Check sheet for the modelled part. Datum: model origin and axes. Units: mm. Coordinates: 2 decimals unless noted, no trailing zeros. Write each loop counter-clockwise with the first axis right and the second up, starting at its lowest first coordinate (ties: lowest second). Pieces come first, ordered by that corner, then holes. Notation, with made-up numbers: M 38.5,35.5 L 45.5,35.5 A20 cw 45.5,71.5 Z; hole C -18,-19 d10. An arc over 180 degrees is marked long. Answer as CSV lines item,"result". Start each with the question number.
Q1. Sectioned sample at D-D, the plane y = 46. Record the cut outline in (x, z), then the cut area to 3 significant figures.
Q2. Sectioned sample at A-A, the plane z = -1.05. Count the separate pieces of the cut face and the enclosed holes in it, then the cut area to 3 significant figures.
Q3. Depth check by flat-ended pin: pin 1 Ø3.5 at (x, y) = (0, 59.309) entering from +Z. Enter the tip coordinate at first touch or a pass-through.
Q4. Sectioned sample at B-B, the plane x = -1. Record the cut outline in (y, z).
Q5. Sectioned sample at C-C, the plane y = -1. Record the cut outline in (x, z), then the cut area to 3 significant figures.
Q6. Thickness scan on line 1 along Y through (x, z) = (0, 0.75) (3 decimals); line 2 along X through (y, z) = (72, -0.1); line 3 along Y through (x, z) = (-0.75, -0.4). Record the ranges inside material, lowest first. Write a range as from..to.
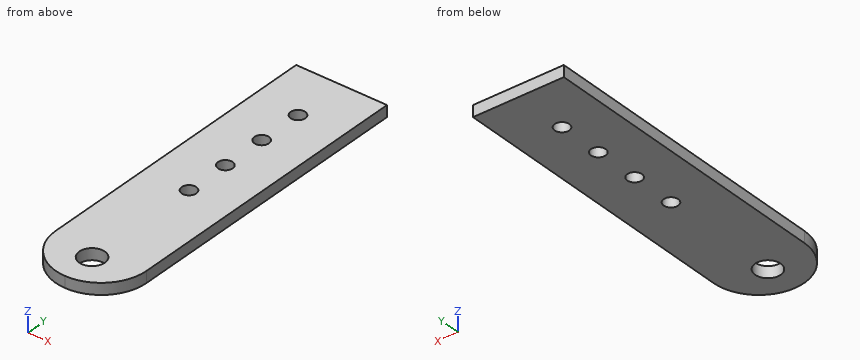
Autodesk Inventor part; units mm, degrees
ref_plane "YZ Plane" through (0, 0, 0) normal (1, 0, 0) x (0, 1, 0)
ref_plane "XZ Plane" through (0, 0, 0) normal (0, 1, 0) x (-1, 0, 0)
ref_plane "XY Plane" through (0, 0, 0) normal (0, 0, 1) x (1, 0, 0)
sketch "Sketch1" plane through (0, 0, 0) normal (0, 0, 1) x (1, 0, 0)
  circle A0 centre (0, 0) radius 3.5687
  line L0 (-12.7, 61.849) -> (12.7, 61.849)
  line L1 (12.7, 61.849) -> (12.7, -9.525)
  line L2 (12.7, -9.525) -> (-12.7, -9.525)
  line L3 (-12.7, -9.525) -> (-12.7, 61.849)
  dimension "d0" = 7.1374
  dimension "d1" = 12.7
  dimension "d2" = 25.4
  dimension "d3" = 9.525
  dimension "d4" = 71.374
extrude "Extrusion1" add sketch "Sketch1" along normal mid plane 3.175
sketch "Sketch2" plane through (0, 0, 1.5875) normal (0, 0, 1) x (1, 0, 0)
  line L0 (-12.7, -9.525) -> (12.7, -9.525)
  point P0 (0, 46.609)
  point P1 (0, 33.909)
  point P2 (0, 59.309)
  point P3 (0, 72.009)
  dimension "d8" = 12.7
  dimension "d20" = 12.7
  dimension "d30" = 12.7
  dimension "d31" = 43.434
hole "Hole1" at (0, 46.609, 1.5875) at (0, 33.909, 1.5875) direction (0, 0, -1) diameter 4.0894 end through all
fillet "Fillet2" radius 12.7 2 edges at (12.7, -9.525, 0) (-12.7, -9.525, 0)
sketch "Sketch3" plane through (-12.7, 61.849, 1.5875) normal (0, 1, 0) x (1, 0, 0)
  line L0 (0, 3.175) -> (0, 0)
  line L1 (25.4, 0) -> (0, 0)
  line L2 (25.4, 0) -> (25.4, 3.175)
  line L3 (0, 3.175) -> (25.4, 3.175)
  point P0 (12.7, 1.5875)
extrude "Extrusion2" add sketch "Sketch3" along normal blind 25.4
hole "Hole2" at (0, 59.309, 1.5875) at (0, 72.009, 1.5875) direction (0, 0, -1) diameter 4.0894 end through all
properties part number "C18_TK_ClimberingSupportGusset" material "Aluminum 6061"
Output:
1,outline,"M -12.7,-1.59 L -1.95,-1.59 L -1.95,1.59 L -12.7,1.59 Z; M 1.95,-1.59 L 12.7,-1.59 L 12.7,1.59 L 1.95,1.59 Z"
1,area,"68.3 mm^2"
2,separate pieces,"1"
2,enclosed holes,"5"
2,area,"2,300 mm^2"
3,pin 1,"passes through"
4,outline,"M -9.49,-1.59 L -3.43,-1.59 L -3.43,1.59 L -9.49,1.59 Z; M 3.43,-1.59 L 32.13,-1.59 L 32.13,1.59 L 3.43,1.59 Z; M 35.69,-1.59 L 44.83,-1.59 L 44.83,1.59 L 35.69,1.59 Z; M 48.39,-1.59 L 57.53,-1.59 L 57.53,1.59 L 48.39,1.59 Z; M 61.09,-1.59 L 70.23,-1.59 L 70.23,1.59 L 61.09,1.59 Z; M 73.79,-1.59 L 87.25,-1.59 L 87.25,1.59 L 73.79,1.59 Z"
5,outline,"M -11.99,-1.59 L -3.43,-1.59 L -3.43,1.59 L -11.99,1.59 Z; M 3.43,-1.59 L 11.99,-1.59 L 11.99,1.59 L 3.43,1.59 Z"
5,area,"54.4 mm^2"
6,line 1,"y = -9.525..-3.569, 3.569..31.864, 35.954..44.564, 48.654..57.264, 61.354..69.964, 74.054..87.249"
6,line 2,"x = -12.7..-2.04, 2.04..12.7"
6,line 3,"y = -9.5..-3.49, 3.49..32.01, 35.81..44.71, 48.51..57.41, 61.21..70.11, 73.91..87.25"
